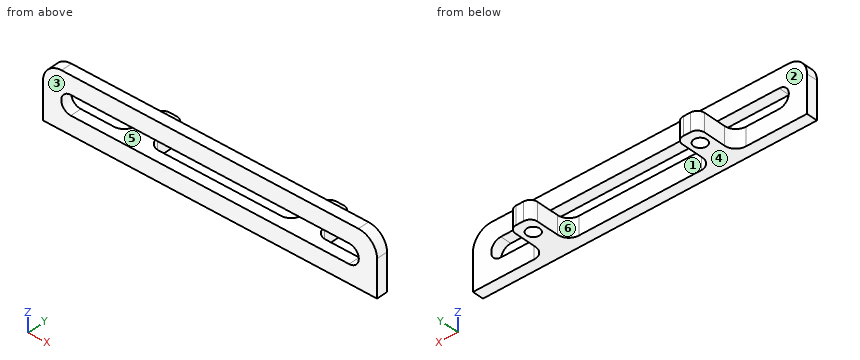
```python
from build123d import *

# Parameters (mm, degrees)
SKETCH1_W           = 90
SKETCH1_H           = 15
BOSS_EXTRUDE1_DEPTH = 3
FILLET1_R           = 5
SKETCH2_W           = 6
SKETCH2_H           = 4.913709841
BOSS_EXTRUDE2_DEPTH = 11
SKETCH3_R           = 1.75
CUT_EXTRUDE1_DEPTH  = 4.913709841
FILLET2_R           = 2
FILLET3_R           = 3


with BuildPart() as part:
    # Sketch1 → Boss-Extrude1 (new body)
    with BuildSketch(Plane(origin=(0, 0, 0), x_dir=(1, 0, 0), z_dir=(0, 1, 0))):
        Rectangle(SKETCH1_W, SKETCH1_H)
        with BuildLine():
            Line((-37.5, 2.586290159), (37.5, 2.586290159))
            ThreePointArc((37.5, 2.586290159), (40.086290159, 0), (37.5, -2.586290159))
            Line((37.5, -2.586290159), (-37.5, -2.586290159))
            ThreePointArc((-37.5, -2.586290159), (-40.086290159, 0), (-37.5, 2.586290159))
        make_face(mode=Mode.SUBTRACT)
    extrude(amount=BOSS_EXTRUDE1_DEPTH)

    # Fillet1
    fillet1_edges = [part.edges().sort_by_distance(p)[0] for p in [
        (45, 1.5, 7.5),
        (-45, 1.5, 7.5),
    ]]
    fillet(fillet1_edges, radius=FILLET1_R)

    # Sketch2 → Boss-Extrude2 (add)
    with BuildSketch(Plane(origin=(0, 3, 0), x_dir=(1, 0, 0), z_dir=(0, 1, 0))):
        with Locations((-22.5, 5.04314508)):
            Rectangle(SKETCH2_W, SKETCH2_H)
        with Locations((22.5, 5.04314508)):
            Rectangle(SKETCH2_W, SKETCH2_H)
    extrude(amount=BOSS_EXTRUDE2_DEPTH)

    # Sketch3 → Cut-Extrude1 (cut)
    with BuildSketch(Plane.XY.offset(-2.586290159)):
        with Locations((-22.5, 10)):
            Circle(SKETCH3_R)
    cut_extrude1 = extrude(amount=-CUT_EXTRUDE1_DEPTH, mode=Mode.SUBTRACT)

    # Mirror1: Cut-Extrude1 across plane
    add(cut_extrude1.mirror(Plane(origin=(0, 0, 0), x_dir=(0, 0, 1), z_dir=(1, 0, 0))), mode=Mode.SUBTRACT)

    # Fillet2
    fillet2_edges = [part.edges().sort_by_distance(p)[0] for p in [
        (-25.5, 14, -5.043145079),
        (-19.5, 14, -5.043145079),
        (19.5, 14, -5.043145079),
        (25.5, 14, -5.043145079),
    ]]
    fillet(fillet2_edges, radius=FILLET2_R)

    # Fillet3
    fillet3_edges = [part.edges().sort_by_distance(p)[0] for p in [
        (-25.5, 3, -5.043145079),
        (-19.5, 3, -5.043145079),
        (19.5, 3, -5.043145079),
        (25.5, 3, -5.043145079),
    ]]
    fillet(fillet3_edges, radius=FILLET3_R)


solid = part.part
```
The listing builds one solid part. Answer for the finished solid, in the listing's coordinates (mm). Face numbers are marked on the shaded views. A direction names the side the tool comes from. Round coordinates to 2 decimals unless told otherwise and drop trailing zeros. Order: outer loops, then holes, each group sorted by start corner. A loop starts at its lowest first (then second) coordinate and runs counter-clockwise, first axis right, second up. Notation, with made-up numbers: (49, 34) - (75, 34) arc R27 cw to (75, 57) - close; hole circle Ø3 at (49.5, 81.25). An arc over 180 degrees is marked (long way). Put each result on its own line as item: value. Start each with the question number.
(1) Find section C-C (x = 22.5). Give the vertices of the cut face in (y, z).
(2) Given P1, Ø5.5, axis at y = 8, z = -4, coming from the +X side; P2, Ø4, axis at y = 9, z = -4, coming from the -X side; P3, Ø1.5, axis at y = 9, z = -5.5, coming from the +X side, each flat-ended and moving along its own axis, determine where each tip first touches the part or whether it passes through.
(3) Find section A-A (y = 10). Give the vertices of the cut face in (x, z), plus the area to 3 significant figures.
(4) For the marked faces 1, 2 and 3, determine the directions among +Z, -Z, +X, -X, +Y, -Y from which every point of the face is accessible in a straight line to the end or side of a thin tool.
(5) Find section B-B (x = -6). Give the vertices of the cut face in (y, z).
(6) Determine the mould class of the marked faces 4, 5 and 6 for opening direction Z: released by +Z, released by -Z, zero draft, split by the parting line, or undercut.
(7) Find section D-D (z = -3.75). Give the vertices of the cut face in (x, y), plus the area to 3 significant figures.
(8) Straight lines are drawn through the part: probe 1 along Y at (x, z) = (-22.5, -5.7); probe 2 along X at (y, z) = (6, -6); probe 3 along Z at (x, y) = (-27, 1.75). For each, find the intervals that lie inside material, in ascending order. Write a range as from..to.
Reply:
1. outline: (0, -7.5) - (8.25, -7.5) - (8.25, -2.59) - (0, -2.59) - close; (0, 2.59) - (3, 2.59) - (3, 7.5) - (0, 7.5) - close; (11.75, -7.5) - (14, -7.5) - (14, -2.59) - (11.75, -2.59) - close
2. P1: x = 25.6
2. P2: x = -25.5
2. P3: x = 25.5
3. outline: (-25.5, -7.5) - (-24.25, -7.5) - (-24.25, -2.59) - (-25.5, -2.59) - close; (-20.75, -7.5) - (-19.5, -7.5) - (-19.5, -2.59) - (-20.75, -2.59) - close; (19.5, -7.5) - (20.75, -7.5) - (20.75, -2.59) - (19.5, -2.59) - close; (24.25, -7.5) - (25.5, -7.5) - (25.5, -2.59) - (24.25, -2.59) - close
3. area: 24.6 mm^2
4. face 1: +Z, -Z, +Y
4. face 2: +Z, +Y
4. face 3: +Z, -Z, +X, -X, -Y
5. outline: (0, -7.5) - (3, -7.5) - (3, -2.59) - (0, -2.59) - close; (0, 2.59) - (3, 2.59) - (3, 7.5) - (0, 7.5) - close
6. face 4: released by -Z
6. face 5: undercut
6. face 6: zero draft
7. outline: (-45, 0) - (45, 0) - (45, 3) - (28.5, 3) arc R3 cw to (25.5, 6) - (25.5, 12) arc R2 ccw to (23.5, 14) - (21.5, 14) arc R2 ccw to (19.5, 12) - (19.5, 6) arc R3 cw to (16.5, 3) - (-16.5, 3) arc R3 cw to (-19.5, 6) - (-19.5, 12) arc R2 ccw to (-21.5, 14) - (-23.5, 14) arc R2 ccw to (-25.5, 12) - (-25.5, 6) arc R3 cw to (-28.5, 3) - (-45, 3) - close; hole circle Ø3.5 at (-22.5, 10); hole circle Ø3.5 at (22.5, 10)
7. area: 387 mm^2
8. probe 1: 0..8.25, 11.75..14
8. probe 2: -25.5..-19.5, 19.5..25.5
8. probe 3: -7.5..-2.59, 2.59..7.5
